Read the model definition and answer for the solid it produces. Units are mm, in the model's axes. A direction names the side the tool comes from. Give positions to 0.01 mm unless a question says otherwise; leave off trailing zeros. Loops run counter-clockwise (first coordinate to the right, second up) from the corner with the lowest first, then second, coordinate; pieces in that order, holes last.
(1) Find section D-D, the plane z = 6. State how many separate pieces and enclosed holes the cut face has, then the cut area to 3 significant figures.
(2) Which of the six approach directions +Z, -Z, +X, -X, +Y, -Y give full straight-line access (tool end or side, diameter ignored) to faces 1 (the face through (-1.648, 13.324, -5.234)), 2 (the face through (-2.44, 54.49, -0.54)), 3 (the face through (0, 0, 0)), 4 (the face through (-2.44, 1.97, -0.54))?
(3) Determine the mould class of faces 5 (the face through (-2.2, 47, -7.1)), 6 (the face through (-1.656, 4.299, -5.258)), 7 (the face through (8, 36, 8)) for opening direction X: pulls with the +X half, pulls with the -X half, needs draft (parallel to the pull), parting line crosses it, or undercut.
(4) Straight lines are drawn through the part: probe 1 along Z at (x, y) = (5, 44); probe 2 along X at (y, z) = (40, 0); probe 3 along X at (y, z) = (42.25, 0). For each, find the intervals that lie inside material, in ascending order.
(5) Find section C-C, the plane y = 3. Write down the section's boundary in (x, z), then the cut area to 3 significant figures.
(6) Find section A-A, the plane y = 44.5. Write down the section's boundary in (x, z).
(7) Each of these flat-tipped pins is pushed along its axis until it touches: P1, Ø9.5, axis at x = -4.5, z = -2, coming from the -Y side; P2, Ø4, axis at x = 12.5, z = -7, coming from the +Y side; P3, Ø10, axis at y = 37, z = 10.5, coming from the -X side; P4, Ø1, axis at x = 2.5, y = 12, coming from the +Z side. Where does it stop, or does it pass through?
(8) Find section B-B, the plane z = -8. Write down the section's boundary in (x, y), then the cut area to 3 significant figures.
```python
from build123d import *

# Parameters (mm, degrees)
SK_P02_GUIDEBOLTDROOPSTOP_R  = 2.5
P02_GUIDEBOLTDROOPSTOP_DEPTH = 55
P04_STOPNUT_START            = 50
SK_P04_STOPNUT_R             = 4.5
P04_STOPNUT_DEPTH            = 4


with BuildPart() as part:
    # SK_P01_Spring → P01_Spring (revolve)
    with BuildSketch(Plane.XY, mode=Mode.PRIVATE) as p01_spring_sk:
        Polygon((0, 4), (5.4, 4), (7.2, 8.778), (5.4, 13.556), (7.2, 18.333), (5.4, 23.111), (7.2, 27.889), (5.4, 32.667), (7.2, 37.444), (5.4, 42.222), (7.2, 47), (0, 47), align=None)
    revolve(p01_spring_sk.sketch.rotate(Axis((0, -1, 0), (0, 1, 0)), 90), axis=Axis((0, -1, 0), (0, 1, 0)))

    # SK_P02_Guideboltdroopstop → P02_Guideboltdroopstop (add)
    with BuildSketch(Plane(origin=(0, 0, 0), x_dir=(1, 0, 0), z_dir=(0, 1, 0))):
        with Locations(Location((0, 0, 0), (0, 0, 270))):
            Circle(SK_P02_GUIDEBOLTDROOPSTOP_R)
    extrude(amount=P02_GUIDEBOLTDROOPSTOP_DEPTH)

    # SK_P03_Springcup → P03_Springcup (revolve)
    with BuildSketch(Plane.XY, mode=Mode.PRIVATE) as p03_springcup_sk:
        Polygon((9.5, 36), (17.5, 36), (17.5, 38), (13, 38), (13, 50), (0, 50), (0, 47), (9.5, 47), align=None)
    revolve(p03_springcup_sk.sketch.rotate(Axis((0, 31, 0), (0, 1, 0)), 90), axis=Axis((0, 31, 0), (0, 1, 0)))

    # SK_P04_Stopnut → P04_Stopnut (add)
    with BuildSketch(Plane(origin=(0, 0, 0), x_dir=(1, 0, 0), z_dir=(0, 1, 0)).offset(P04_STOPNUT_START)):
        with Locations(Location((0, 0, 0), (0, 0, 270))):
            Circle(SK_P04_STOPNUT_R)
    extrude(amount=P04_STOPNUT_DEPTH)


solid = part.part
```
Entries:
1. separate pieces: 5
1. enclosed holes: 0
1. area: 330 mm2
2. face 1: none
2. face 2: +Y
2. face 3: +Z, -Z, +X, -X, -Y
2. face 4: -Y
3. face 5: undercut
3. face 6: parting line crosses it
3. face 7: needs draft
4. probe 1: z = -12 to -8.08, -3.44 to 3.44, 8.08 to 12
4. probe 2: x = -13 to -9.5, -6.24 to 6.24, 9.5 to 13
4. probe 3: x = -13 to -9.5, -5.41 to 5.41, 9.5 to 13
5. outline: circle Ø5 at (0, 0)
5. area: 19.6 mm2
6. outline: circle Ø26 at (0, 0); circle Ø12.52 at (0, 0); hole circle Ø19 at (0, 0)
7. P1: stops at y = 0
7. P2: stops at y = 50
7. P3: stops at x = -16.61
7. P4: stops at z = 5.73
8. outline: (-15.56, 36) - (-5.12, 36) - (-5.12, 47) - (5.12, 47) - (5.12, 36) - (15.56, 36) - (15.56, 38) - (10.25, 38) - (10.25, 50) - (-10.25, 50) - (-10.25, 38) - (-15.56, 38) - close
8. area: 195 mm2
